The listing builds one solid part. Answer for the finished solid, in the listing's coordinates (mm). Coordinates: 2 decimals unless noted, no trailing zeros. Order: outer loops, then holes, each group sorted by start corner. A loop starts at its lowest first (then second) coordinate and runs counter-clockwise, first axis right, second up. Notation, with made-up numbers: (-0.5, 0.5) -> (42.5, 0.5) arc R15 ccw to (42.5, 17.5) -> close; hole circle Ø9 at (57, 57.5). An arc over 180 degrees is marked (long way). Answer in a Markdown table with one row per item. Add a question column.
```python
from build123d import *

# Parameters (mm, degrees)
SKETCH1_W           = 7
SKETCH1_H           = 42
SKETCH1_W_2         = 40
SKETCH1_H_2         = 6
BOSS_EXTRUDE1_DEPTH = 6


with BuildPart() as part:
    # Sketch1 → Boss-Extrude1 (new body)
    with BuildSketch(Plane(origin=(0, 0, 0), x_dir=(0, 0, -1), z_dir=(1, 0, 0))):
        Polygon((-46.246943765, 21.420537897), (-20.246943765, 21.420537897), (-20.246943765, 24.420537897), (5.753056235, 24.420537897), (5.753056235, 21.420537897), (31.753056235, 21.420537897), (31.753056235, 24.420537897), (57.753056235, 24.420537897), (57.753056235, 21.420537897), (83.753056235, 21.420537897), (83.753056235, 7.420537897), (89.753056235, 7.420537897), (89.753056235, -12.579462103), (83.753056235, -12.579462103), (83.753056235, -32.579462103), (57.753056235, -32.579462103), (57.753056235, -38.579462103), (31.753056235, -38.579462103), (31.753056235, -32.579462103), (5.753056235, -32.579462103), (5.753056235, -38.579462103), (-20.246943765, -38.579462103), (-20.246943765, -32.579462103), (-46.246943765, -32.579462103), (-46.246943765, -12.579462103), (-52.246943765, -12.579462103), (-52.246943765, 7.420537897), (-46.246943765, 7.420537897), align=None)
        with Locations((-36.746943765, -5.579462103)):
            Rectangle(SKETCH1_W, SKETCH1_H, mode=Mode.SUBTRACT)
        with Locations((48.253056235, -5.579462103)):
            Rectangle(SKETCH1_W, SKETCH1_H, mode=Mode.SUBTRACT)
        with Locations((-23.746943765, -5.579462103)):
            Rectangle(SKETCH1_W, SKETCH1_H, mode=Mode.SUBTRACT)
        with Locations((-10.746943765, -5.579462103)):
            Rectangle(SKETCH1_W, SKETCH1_H, mode=Mode.SUBTRACT)
        with Locations((18.753056235, -23.579462103)):
            Rectangle(SKETCH1_W_2, SKETCH1_H_2, mode=Mode.SUBTRACT)
        with Locations((61.253056235, -5.579462103)):
            Rectangle(SKETCH1_W, SKETCH1_H, mode=Mode.SUBTRACT)
        with Locations((74.253056235, -5.579462103)):
            Rectangle(SKETCH1_W, SKETCH1_H, mode=Mode.SUBTRACT)
    extrude(amount=BOSS_EXTRUDE1_DEPTH)


solid = part.part
```
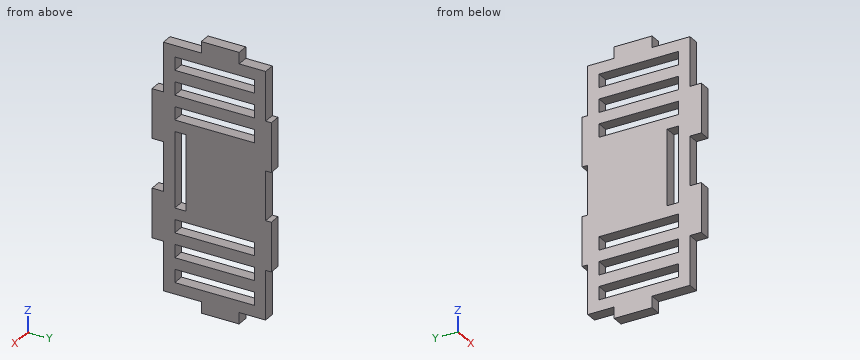
Q1. A cutting plane is placed at C-C (z = -21.5). Determine the outline of the cut face in (x, y), then the cut area to 3 significant figures.
Q2. A cutting plane is placed at D-D (x = 1.6). State how many separate pieces and enclosed holes the cut face has, then the cut area to 3 significant figures.
Q3. Given pin 1 (1.5 mm diameter, centred on x = 4.5, y = 22.5, fed in from -Z); pin 2 (3 mm diameter, centred on x = 1.5, z = -60, fed in from -Y); pin 3 (1 mm diameter, centred on y = -21.5, z = -32.5, fed in from +X); pin 4 (1.8 mm diameter, centred on x = 3, z = 37.5, fed in from +Y), each flat-ended and moving along its own axis, determine where each tip first touches the part or whether it passes through.
Q4. A cutting plane is placed at A-A (z = 22.5). Determine the outline of the cut face in (x, y).
Q5. A cutting plane is placed at B-B (y = 3.5). Determine the outline of the cut face in (x, z), then the cut area to 3 significant figures.
Q6. Straight lines are drawn through the part: line 1 (Y direction, x = 5.05, z = -74); line 2 (Z direction, x = 4.4, y = -34); line 3 (Y direction, x = 0.85, z = -11.5). For each, find the intervals that lie inside material, in ascending order.
Returned:
| question | item | result |
|---|---|---|
| 1 | outline | (0, -32.58) -> (6, -32.58) -> (6, -26.58) -> (0, -26.58) -> close; (0, -20.58) -> (6, -20.58) -> (6, 21.42) -> (0, 21.42) -> close |
| 1 | area | 288 mm² |
| 2 | separate pieces | 1 |
| 2 | enclosed holes | 7 |
| 2 | area | 5,720 mm² |
| 3 | pin 1 | stops at z = -57.75 |
| 3 | pin 2 | stops at y = -32.58 |
| 3 | pin 3 | passes through |
| 3 | pin 4 | stops at y = 21.42 |
| 4 | outline | (0, -32.58) -> (6, -32.58) -> (6, -26.58) -> (0, -26.58) -> close; (0, 15.42) -> (6, 15.42) -> (6, 21.42) -> (0, 21.42) -> close |
| 5 | outline | (0, -89.75) -> (6, -89.75) -> (6, -77.75) -> (0, -77.75) -> close; (0, -70.75) -> (6, -70.75) -> (6, -64.75) -> (0, -64.75) -> close; (0, -57.75) -> (6, -57.75) -> (6, -51.75) -> (0, -51.75) -> close; (0, -44.75) -> (6, -44.75) -> (6, 7.25) -> (0, 7.25) -> close; (0, 14.25) -> (6, 14.25) -> (6, 20.25) -> (0, 20.25) -> close; (0, 27.25) -> (6, 27.25) -> (6, 33.25) -> (0, 33.25) -> close; (0, 40.25) -> (6, 40.25) -> (6, 52.25) -> (0, 52.25) -> close |
| 5 | area | 600 mm² |
| 6 | line 1 | y = -32.58 to -26.58, 15.42 to 21.42 |
| 6 | line 2 | z = -57.75 to -31.75, -5.75 to 20.25 |
| 6 | line 3 | y = -32.58 to -26.58, -20.58 to 21.42 |
